The model under review builds one solid part; all positions refer to its coordinate system, in mm. A direction names the side the tool comes from. Round coordinates to 2 decimals unless told otherwise and drop trailing zeros. Order: outer loops, then holes, each group sorted by start corner. A loop starts at its lowest first (then second) coordinate and runs counter-clockwise, first axis right, second up. Notation, with made-up numbers: M -3,61 L 12,61 A21 ccw 12,81 Z; hole C 61,12 d4. An arc over 180 degrees is marked long. Answer as a JSON object with one key per item and string values. Group by question number.
1. Mouldability with a two-part tool opening along Y and no side actions: class faces 5 (the face through (14.24, -45.73, 25.35)), 6 (the face through (7, -20, 15)), 7 (the face through (15.5, -24.6, 50)) as released by +Y, released by -Y, zero draft, split by the parting line, or undercut.
2. Add section D-D on y = -21. State the section outline as (x, z) points, and give its area (3 significant figures).
3. Clearance check with flat-ended pins moving along their axes: P1, Ø4, axis at x = 43.5, z = 19.5, coming from the +Y side; P2, Ø5, axis at x = 16, z = 10, coming from the -Y side; P3, Ø1, axis at x = 34.5, y = -33, coming from the +Z side. State where each tip first meets the part, or that it passes through.
4. To check wall thickness, follow probe 1 along Z at (x, y) = (20, -25); probe 2 along Y at (x, z) = (5, 15); probe 3 along X at (y, z) = (-33, 21.5). State the ranges of each line that lie inside material, in increasing order. Write a range as [from, to].
5. Add section C-C on z = 32.5. State the section outline as (x, y) points, and give its area (3 significant figures).
6. Machinability: for faces 1 (the face through (15, -25, 25)), 2 (the face through (15, -25, 8)), 3 (the face through (25, -25, 43)), 4 (the face through (7, -30, 45)), which of the approach directions +Z, -Z, +X, -X, +Y, -Y give a long, thin tool a straight path to every point of the face, cutting with its end or side? Answer none if there is none.
7. Add section A-A on x = 18. State the section outline as (y, z) points.
8. Add section B-B on x = 4.5. State the section outline as (y, z) points.
```python
from build123d import *

# Parameters (mm, degrees)
F1_DEPTH = 50
F3_DEPTH = 15
F6_DEPTH = 50


with BuildPart() as f1:
    # F0 (on Front) → F1 (new body)
    with BuildSketch(Plane.XZ):
        with BuildLine():
            Line((25, 50), (0, 50))
            Line((0, 50), (0, 0))
            Line((0, 0), (25, 0))
            ThreePointArc((25, 0), (42.6776695297, 7.3223304703), (50, 25))
            ThreePointArc((50, 25), (42.6776695297, 42.6776695297), (25, 50))
        make_face()
        with BuildLine():
            Line((25, 15), (15, 15))
            Line((15, 15), (15, 35))
            Line((15, 35), (25, 35))
            ThreePointArc((25, 35), (32.0710678119, 32.0710678119), (35, 25))
            ThreePointArc((35, 25), (32.0710678119, 17.9289321881), (25, 15))
        make_face(mode=Mode.SUBTRACT)
    extrude(amount=F1_DEPTH)

    # F2 (on face) → F3 (cut)
    with BuildSketch(Plane(origin=(0, 0, 0), x_dir=(0, -1, 0), z_dir=(-1, 0, 0))):
        Polygon((15, 20), (15, 0), (35, 0), (35, 20), (25, 10), align=None)
        Polygon((35, 50), (15, 50), (25, 40), align=None)
    extrude(amount=-F3_DEPTH, mode=Mode.SUBTRACT)

    # F5 (on offset) → F6 (cut)
    with BuildSketch(Plane.XY.offset(50)):
        Polygon((41.6666666667, -25), (25, -20), (25, -30), align=None)
        Polygon((50, -50), (50, -35), (0, -50), align=None)
        Polygon((0, 0), (50, -15), (50, 0), align=None)
    extrude(amount=-F6_DEPTH, mode=Mode.SUBTRACT)


solid = f1.part
```
Recorded:
{
 "1": {"face 5": "released by -Y", "face 6": "undercut", "face 7": "zero draft"},
 "2": {"outline": "M 0,14 L 15,14 L 15,0 L 25,0 L 25,15 L 15,15 L 15,35 L 25,35 L 25,50 L 15,50 L 15,44 L 0,44 Z; M 28.33,0.22 A25 ccw 28.33,49.78 L 28.33,34.43 A10 cw 28.33,15.57 Z", "area": "1,470 mm²"},
 "3": {"P1": "stops at y = -12.45", "P2": "stops at y = -45.95", "P3": "stops at z = 48.32"},
 "4": {"probe 1": "z = [0, 15], [35, 50]", "probe 2": "y = [-48.5, -35], [-30, -20], [-15, -1.5]", "probe 3": "x = [0, 15], [34.37, 49.75]"},
 "5": {"outline": "M 0,-50 L 15,-45.5 L 15,-4.5 L 0,0 Z; M 31.61,-40.52 L 48.85,-35.35 L 48.85,-14.65 L 31.61,-9.48 L 31.61,-21.98 L 41.67,-25 L 31.61,-28.02 Z", "area": "1,100 mm²"},
 "6": {"face 1": "+Y, -Y", "face 2": "-Z, -X", "face 3": "+Z, -Z", "face 4": "+Z, -X"},
 "7": {"outline": "M -44.6,0 L -5.4,0 L -5.4,15 L -44.6,15 Z; M -44.6,35 L -5.4,35 L -5.4,50 L -44.6,50 Z"},
 "8": {"outline": "M -48.65,0 L -35,0 L -35,20 L -25,10 L -15,20 L -15,0 L -1.35,0 L -1.35,50 L -15,50 L -25,40 L -35,50 L -48.65,50 Z"}
}
